Geometry check sheet. Reference: drawing and pictorial views, mm from the part's lowest x, y, z. Give positions to 0.01 mm unless a question says otherwise; leave off trailing zeros. Loops run counter-clockwise (first coordinate to the right, second up) from the corner with the lowest first, then second, coordinate; pieces in that order, holes last. Notation, with made-up numbers: (45.25, -9) - (86.25, -9) arc R9 cw to (86.25, -5) - close; hole circle Ø5 at (-16, 11.5). An arc over 180 degrees is marked (long way). Put each result on its own line as item: value. Start each with the question number.
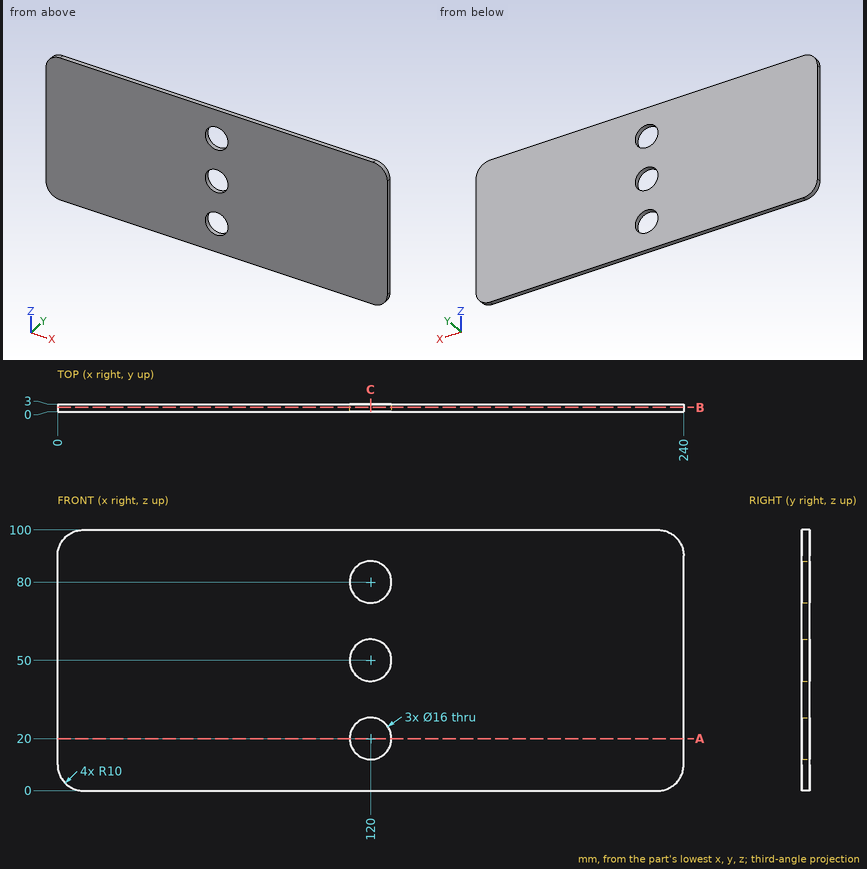
1) Scan lines: line 1 along Z through (x, y) = (120, 1.7); line 2 along Z through (x, y) = (126, 1.35). Record each from-to range of solid material in increasing order. Write a range as from..to.
2) Section check C-C, the plane x = 120. Enter the section's corners in (y, z).
3) Depth check by flat-ended pin: P1, Ø13, axis at x = 120, z = 20, coming from the -Y side. Enter the tip coordinate at first touch or a pass-through.
4) Section check B-B, the plane y = 1.7. Enter the section's corners in (x, z).
5) Section check A-A, the plane z = 20. Enter the section's corners in (x, y), plus the area to 3 significant figures.
Results are:
1. line 1: z = 0..12, 28..42, 58..72, 88..100
1. line 2: z = 0..14.71, 25.29..44.71, 55.29..74.71, 85.29..100
2. outline: (0, 0) - (3, 0) - (3, 12) - (0, 12) - close; (0, 28) - (3, 28) - (3, 42) - (0, 42) - close; (0, 58) - (3, 58) - (3, 72) - (0, 72) - close; (0, 88) - (3, 88) - (3, 100) - (0, 100) - close
3. P1: passes through
4. outline: (0, 10) arc R10 ccw to (10, 0) - (230, 0) arc R10 ccw to (240, 10) - (240, 90) arc R10 ccw to (230, 100) - (10, 100) arc R10 ccw to (0, 90) - close; hole circle Ø16 at (120, 20); hole circle Ø16 at (120, 50); hole circle Ø16 at (120, 80)
5. outline: (0, 0) - (112, 0) - (112, 3) - (0, 3) - close; (128, 0) - (240, 0) - (240, 3) - (128, 3) - close
5. area: 672 mm2
